For this review, take the finished solid that the model builds, in its own axes (mm). Face numbers are marked on the shaded views. Round coordinates to 2 decimals unless told otherwise and drop trailing zeros. Write each loop counter-clockwise with the first axis right and the second up, starting at its lowest first coordinate (ties: lowest second). Pieces come first, ordered by that corner, then holes.
Autodesk Inventor part; units mm, degrees
ref_plane "YZ Plane" through (0, 0, 0) normal (1, 0, 0) x (0, 1, 0)
ref_plane "XZ Plane" through (0, 0, 0) normal (0, 1, 0) x (-1, 0, 0)
ref_plane "XY Plane" through (0, 0, 0) normal (0, 0, 1) x (1, 0, 0)
sketch "Sketch1" plane through (0, 0, 0) normal (0, 0, 1) x (1, 0, 0)
  circle A0 centre (0, 0) radius 6.25
  circle A1 centre (0, 0) radius 8
  dimension "d0" = 12.5
  dimension "d1" = 16
extrude "Extrusion1" add sketch "Sketch1" along normal mid plane 52
chamfer "Chamfer1" distance 0.1 angle 45 4 edges at (-6.25, 0, 26) (-8, 0, 26) (-6.25, 0, -26) (-8, 0, -26)
sketch "Sketch2" plane through (0, 0, 26) normal (0, 0, 1) x (1, 0, 0)
  point P0 (0, 0)
sketch "Sketch3" plane through (0, 0, 26) normal (0, 0, 1) x (1, 0, 0)
  circle A0 centre (0, 0) radius 7
  dimension "d7" = 14
extrude "Extrusion2" cut sketch "Sketch3" against normal blind 10
sketch "Sketch4" plane through (0, 0, -26) normal (0, 0, -1) x (-1, 0, 0)
  circle A0 centre (0, 0) radius 7
  dimension "d10" = 14
extrude "Extrusion3" cut sketch "Sketch4" against normal blind 9.8
properties part number "Joint1_Hand_Bushing"
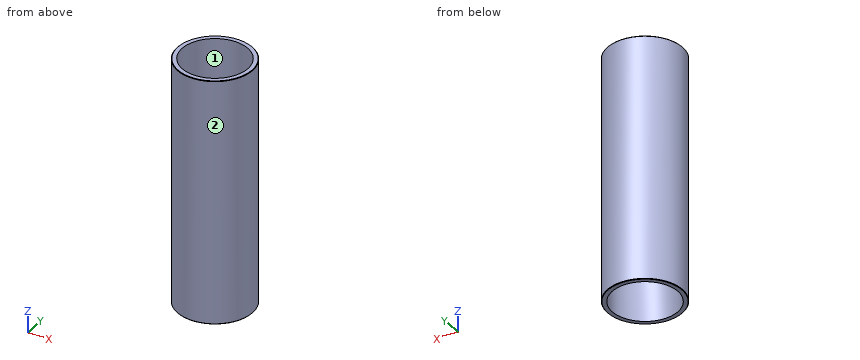
(1) Mouldability with a two-part tool opening along X and no side actions: class the marked faces 1 and 2 as pulls with the +X half, pulls with the -X half, needs draft (parallel to the pull), parting line crosses it, or undercut.
Geometry check:
face 1: undercut
face 2: parting line crosses it
(2) For line 1 along X through (y, z) = (0.25, -14) (3 decimals); line 2 along Y through (x, z) = (0, 19.25); line 3 along X through (y, z) = (5.75, -5.5), list the stretches that pass through material, from the lowest coordinate up.
Geometry check:
line 1: x = -7.996 to -6.245, 6.245 to 7.996
line 2: y = -8 to -7, 7 to 8
line 3: x = -5.56 to -2.45, 2.45 to 5.56
(3) We need section D-D, the plane z = 17. Give the boundary of the cut face in (x, y).
Geometry check:
outline: circle Ø16 at (0, 0); hole circle Ø14 at (0, 0)
(4) We need section A-A, the plane x = 0. Give the boundary of the cut face in (y, z).
Geometry check:
outline: (-8, -25.9) - (-7.9, -26) - (-7, -26) - (-7, -16.2) - (-6.25, -16.2) - (-6.25, 16) - (-7, 16) - (-7, 26) - (-7.9, 26) - (-8, 25.9) - close; (6.25, -16.2) - (7, -16.2) - (7, -26) - (7.9, -26) - (8, -25.9) - (8, 25.9) - (7.9, 26) - (7, 26) - (7, 16) - (6.25, 16) - close
(5) For pin 1 Ø8 at (x, z) = (6, -13) entering from +Y; pin 2 Ø7.5 at (x, y) = (0, 0) entering from -Z; pin 3 Ø3 at (y, z) = (5, -3.5) entering from -X; pin 4 Ø1 at (y, z) = (4.5, -16) entering from -X, all flat-tipped, find the tip position at first contact; note any pin that passes through.
Geometry check:
pin 1: stops at y = 7.75
pin 2: passes through
pin 3: stops at x = -7.19
pin 4: stops at x = -6.93
(6) We need section C-C, the plane z = -14.5. Give the boundary of the cut face in (x, y).
Geometry check:
outline: circle Ø16 at (0, 0); hole circle Ø12.5 at (0, 0)
